Design review of the part built by this model. Coordinates are the model's own, in mm. Give positions to 0.01 mm unless a question says otherwise; leave off trailing zeros. Loops run counter-clockwise (first coordinate to the right, second up) from the corner with the lowest first, then second, coordinate; pieces in that order, holes last. Notation, with made-up numbers: (51.25, 12) - (60.25, 12) arc R12 ccw to (60.25, 32) - close; hole circle Ø9 at (-22, 20.25). An arc over 180 degrees is marked (long way). One line per item, written item: value. Start each with the question number.
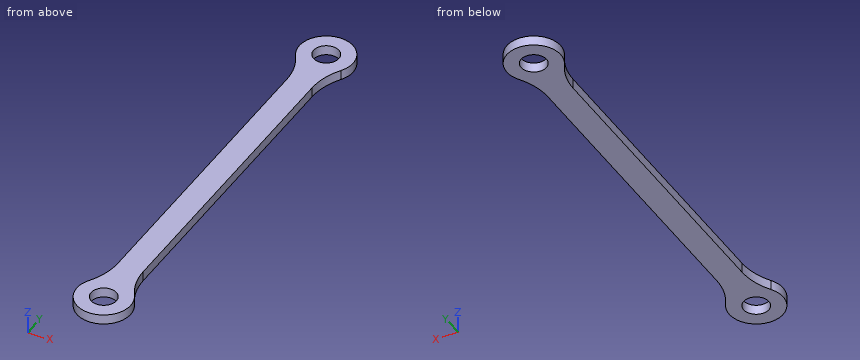
```python
from build123d import *

# Parameters (mm, degrees)
SKETCH1_R           = 8
BOSS_EXTRUDE1_DEPTH = 6.2


with BuildPart() as part:
    # Sketch1 → Boss-Extrude1 (new body)
    with BuildSketch(Plane.XY):
        with BuildLine():
            Line((-8, 96.851957648), (-8, -96.851957648))
            ThreePointArc((-8, -96.851957648), (-9.603702256, -108.064643302), (-14.286215979, -118.378238492))
            ThreePointArc((-14.286215979, -118.378238492), (0, -144.45), (14.286215979, -118.378238492))
            ThreePointArc((14.286215979, -118.378238492), (9.603702256, -108.064643302), (8, -96.851957648))
            Line((8, -96.851957648), (8, 96.851957648))
            ThreePointArc((8, 96.851957648), (9.603702256, 108.064643302), (14.286215979, 118.378238492))
            ThreePointArc((14.286215979, 118.378238492), (0, 144.45), (-14.286215979, 118.378238492))
            ThreePointArc((-14.286215979, 118.378238492), (-9.603702256, 108.064643302), (-8, 96.851957648))
        make_face()
        with Locations(Location((0, 127.5, 0), (0, 0, 180))):
            Circle(SKETCH1_R, mode=Mode.SUBTRACT)
        with Locations(Location((0, -127.5, 0), (0, 0, 180))):
            Circle(SKETCH1_R, mode=Mode.SUBTRACT)
    extrude(amount=BOSS_EXTRUDE1_DEPTH)


solid = part.part
```
(1) To check wall thickness, follow L1, parallel to Y at x = 0, z = 4.5; L2, parallel to X at y = 127.5, z = 1.5; L3, parallel to Y at x = -4, z = 2. State the ranges of each line that lie inside material, in increasing order. Write a range as from..to.
(2) Take a section at B-B on x = 0. State the section outline as (y, z) points.
(3) Take a section at A-A on y = 127.5. State the section outline as (x, z) points, and give its area (3 significant figures).
(4) Take a section at D-D on y = -42.5. State the section outline as (x, z) points.
(5) Take a section at C-C on z = 5.25. State the section outline as (x, y) points.
(6) For pin 1 Ø14.5 at (x, y) = (0, 127.5) entering from +Z; pin 2 Ø3 at (y, z) = (-92, 1) entering from -X; pin 3 Ø1.5 at (x, z) = (-6.5, 3.5) entering from -Y; pin 4 Ø1.5 at (y, z) = (9.5, 2) entering from +X, all flat-tipped, find the tip position at first contact; note any pin that passes through.
Here are the results:
1. L1: -144.45..-135.5, -119.5..119.5, 135.5..144.45
1. L2: -16.95..-8, 8..16.95
1. L3: -143.97..-134.43, -120.57..120.57, 134.43..143.97
2. outline: (-144.45, 0) - (-135.5, 0) - (-135.5, 6.2) - (-144.45, 6.2) - close; (-119.5, 0) - (119.5, 0) - (119.5, 6.2) - (-119.5, 6.2) - close; (135.5, 0) - (144.45, 0) - (144.45, 6.2) - (135.5, 6.2) - close
3. outline: (-16.95, 0) - (-8, 0) - (-8, 6.2) - (-16.95, 6.2) - close; (8, 0) - (16.95, 0) - (16.95, 6.2) - (8, 6.2) - close
3. area: 111 mm²
4. outline: (-8, 0) - (8, 0) - (8, 6.2) - (-8, 6.2) - close
5. outline: (-14.29, -118.38) arc R16.95 ccw (long way) to (14.29, -118.38) arc R40 cw to (8, -96.85) - (8, 96.85) arc R40 cw to (14.29, 118.38) arc R16.95 ccw (long way) to (-14.29, 118.38) arc R40 cw to (-8, 96.85) - (-8, -96.85) arc R40 cw to start; hole circle Ø16 at (0, -127.5); hole circle Ø16 at (0, 127.5)
6. pin 1: through
6. pin 2: x = -8
6. pin 3: y = -143.44
6. pin 4: x = 8
